```python
from build123d import *

# Parameters (mm, degrees)
SKETCH1_W           = 148
SKETCH1_H           = 106
BOSS_EXTRUDE1_DEPTH = 8
CUT_EXTRUDE1_REACH  = 93.373
SKETCH3_R           = 1.65
CUT_EXTRUDE2_DEPTH  = 130.52219887
SKETCH5_R           = 1.65
CUT_EXTRUDE3_DEPTH  = 10
SKETCH6_R           = 1.65
CUT_EXTRUDE4_DEPTH  = 10


with BuildPart() as part:
    # Sketch1 → Boss-Extrude1 (new body)
    with BuildSketch(Plane.XY):
        Rectangle(SKETCH1_W, SKETCH1_H)
    extrude(amount=-BOSS_EXTRUDE1_DEPTH)

    # Sketch2 → Cut-Extrude1 (cut, up to next)
    with BuildSketch(Plane.XY, mode=Mode.PRIVATE) as cut_extrude1_sk1:
        with BuildLine():
            ThreePointArc((60.25, 33.75), (59.373475383, 36.872498999), (57, 39.082682252))
            Line((57, 39.082682252), (57, -39.082682252))
            ThreePointArc((57, -39.082682252), (59.373475383, -36.872498999), (60.25, -33.75))
            Line((60.25, -33.75), (60.25, 33.75))
        make_face()
    cut_extrude1_tool1 = extrude(cut_extrude1_sk1.sketch, amount=-CUT_EXTRUDE1_REACH, mode=Mode.PRIVATE) & part.part
    # Sketch2 → Cut-Extrude1 (cut, up to next)
    with BuildSketch(Plane.XY, mode=Mode.PRIVATE) as cut_extrude1_sk2:
        with BuildLine():
            ThreePointArc((-54.25, 39.75), (-55.66490397, 39.580784403), (-57, 39.082682252))
            Line((-57, 39.082682252), (-57, -39.082682252))
            ThreePointArc((-57, -39.082682252), (-55.66490397, -39.580784403), (-54.25, -39.75))
            Line((-54.25, -39.75), (54.25, -39.75))
            ThreePointArc((54.25, -39.75), (55.66490397, -39.580784403), (57, -39.082682252))
            Line((57, -39.082682252), (57, 39.082682252))
            ThreePointArc((57, 39.082682252), (55.66490397, 39.580784403), (54.25, 39.75))
            Line((54.25, 39.75), (-54.25, 39.75))
        make_face()
    cut_extrude1_tool2 = extrude(cut_extrude1_sk2.sketch, amount=-CUT_EXTRUDE1_REACH, mode=Mode.PRIVATE) & part.part
    # Sketch2 → Cut-Extrude1 (cut, up to next)
    with BuildSketch(Plane.XY, mode=Mode.PRIVATE) as cut_extrude1_sk3:
        with BuildLine():
            Line((-57, -39.082682252), (-57, 39.082682252))
            ThreePointArc((-57, 39.082682252), (-59.373475383, 36.872498999), (-60.25, 33.75))
            Line((-60.25, 33.75), (-60.25, -33.75))
            ThreePointArc((-60.25, -33.75), (-59.373475383, -36.872498999), (-57, -39.082682252))
        make_face()
    cut_extrude1_tool3 = extrude(cut_extrude1_sk3.sketch, amount=-CUT_EXTRUDE1_REACH, mode=Mode.PRIVATE) & part.part
    # Sketch2 → Cut-Extrude1 (cut, up to next)
    with BuildSketch(Plane.XY, mode=Mode.PRIVATE) as cut_extrude1_sk4:
        with BuildLine():
            ThreePointArc((59.1, 46), (57, 48.1), (54.9, 46))
            Line((54.9, 46), (57, 46))
            Line((57, 46), (57, 43.9))
            ThreePointArc((57, 43.9), (58.48492424, 44.51507576), (59.1, 46))
        make_face()
    cut_extrude1_tool4 = extrude(cut_extrude1_sk4.sketch, amount=-CUT_EXTRUDE1_REACH, mode=Mode.PRIVATE) & part.part
    # Sketch2 → Cut-Extrude1 (cut, up to next)
    with BuildSketch(Plane.XY, mode=Mode.PRIVATE) as cut_extrude1_sk5:
        with BuildLine():
            Line((57, 46), (54.9, 46))
            ThreePointArc((54.9, 46), (55.51507576, 44.51507576), (57, 43.9))
            Line((57, 43.9), (57, 46))
        make_face()
    cut_extrude1_tool5 = extrude(cut_extrude1_sk5.sketch, amount=-CUT_EXTRUDE1_REACH, mode=Mode.PRIVATE) & part.part
    # Sketch2 → Cut-Extrude1 (cut, up to next)
    with BuildSketch(Plane.XY, mode=Mode.PRIVATE) as cut_extrude1_sk6:
        with BuildLine():
            ThreePointArc((59.1, 46), (57, 48.1), (54.9, 46))
            Line((54.9, 46), (57, 46))
            Line((57, 46), (57, 43.9))
            ThreePointArc((57, 43.9), (58.48492424, 44.51507576), (59.1, 46))
        make_face()
    cut_extrude1_tool6 = extrude(cut_extrude1_sk6.sketch, amount=-CUT_EXTRUDE1_REACH, mode=Mode.PRIVATE) & part.part
    # Sketch2 → Cut-Extrude1 (cut, up to next)
    with BuildSketch(Plane.XY, mode=Mode.PRIVATE) as cut_extrude1_sk7:
        with BuildLine():
            Line((57, 46), (54.9, 46))
            ThreePointArc((54.9, 46), (55.51507576, 44.51507576), (57, 43.9))
            Line((57, 43.9), (57, 46))
        make_face()
    cut_extrude1_tool7 = extrude(cut_extrude1_sk7.sketch, amount=-CUT_EXTRUDE1_REACH, mode=Mode.PRIVATE) & part.part
    # Sketch2 → Cut-Extrude1 (cut, up to next)
    with BuildSketch(Plane.XY, mode=Mode.PRIVATE) as cut_extrude1_sk8:
        with BuildLine():
            Line((-57, 43.9), (-57, 46))
            Line((-57, 46), (-54.9, 46))
            ThreePointArc((-54.9, 46), (-58.48492424, 47.48492424), (-57, 43.9))
        make_face()
    cut_extrude1_tool8 = extrude(cut_extrude1_sk8.sketch, amount=-CUT_EXTRUDE1_REACH, mode=Mode.PRIVATE) & part.part
    # Sketch2 → Cut-Extrude1 (cut, up to next)
    with BuildSketch(Plane.XY, mode=Mode.PRIVATE) as cut_extrude1_sk9:
        with BuildLine():
            Line((-54.9, 46), (-57, 46))
            Line((-57, 46), (-57, 43.9))
            ThreePointArc((-57, 43.9), (-55.51507576, 44.51507576), (-54.9, 46))
        make_face()
    cut_extrude1_tool9 = extrude(cut_extrude1_sk9.sketch, amount=-CUT_EXTRUDE1_REACH, mode=Mode.PRIVATE) & part.part
    # Sketch2 → Cut-Extrude1 (cut, up to next)
    with BuildSketch(Plane.XY, mode=Mode.PRIVATE) as cut_extrude1_sk10:
        with BuildLine():
            Line((-57, 43.9), (-57, 46))
            Line((-57, 46), (-54.9, 46))
            ThreePointArc((-54.9, 46), (-58.48492424, 47.48492424), (-57, 43.9))
        make_face()
    cut_extrude1_tool10 = extrude(cut_extrude1_sk10.sketch, amount=-CUT_EXTRUDE1_REACH, mode=Mode.PRIVATE) & part.part
    # Sketch2 → Cut-Extrude1 (cut, up to next)
    with BuildSketch(Plane.XY, mode=Mode.PRIVATE) as cut_extrude1_sk11:
        with BuildLine():
            Line((-54.9, 46), (-57, 46))
            Line((-57, 46), (-57, 43.9))
            ThreePointArc((-57, 43.9), (-55.51507576, 44.51507576), (-54.9, 46))
        make_face()
    cut_extrude1_tool11 = extrude(cut_extrude1_sk11.sketch, amount=-CUT_EXTRUDE1_REACH, mode=Mode.PRIVATE) & part.part
    # Sketch2 → Cut-Extrude1 (cut, up to next)
    with BuildSketch(Plane.XY, mode=Mode.PRIVATE) as cut_extrude1_sk12:
        with BuildLine():
            ThreePointArc((-54.9, -46), (-55.51507576, -44.51507576), (-57, -43.9))
            Line((-57, -43.9), (-57, -46))
            Line((-57, -46), (-54.9, -46))
        make_face()
    cut_extrude1_tool12 = extrude(cut_extrude1_sk12.sketch, amount=-CUT_EXTRUDE1_REACH, mode=Mode.PRIVATE) & part.part
    # Sketch2 → Cut-Extrude1 (cut, up to next)
    with BuildSketch(Plane.XY, mode=Mode.PRIVATE) as cut_extrude1_sk13:
        with BuildLine():
            Line((-57, -46), (-57, -43.9))
            ThreePointArc((-57, -43.9), (-58.48492424, -47.48492424), (-54.9, -46))
            Line((-54.9, -46), (-57, -46))
        make_face()
    cut_extrude1_tool13 = extrude(cut_extrude1_sk13.sketch, amount=-CUT_EXTRUDE1_REACH, mode=Mode.PRIVATE) & part.part
    # Sketch2 → Cut-Extrude1 (cut, up to next)
    with BuildSketch(Plane.XY, mode=Mode.PRIVATE) as cut_extrude1_sk14:
        with BuildLine():
            ThreePointArc((-54.9, -46), (-55.51507576, -44.51507576), (-57, -43.9))
            Line((-57, -43.9), (-57, -46))
            Line((-57, -46), (-54.9, -46))
        make_face()
    cut_extrude1_tool14 = extrude(cut_extrude1_sk14.sketch, amount=-CUT_EXTRUDE1_REACH, mode=Mode.PRIVATE) & part.part
    # Sketch2 → Cut-Extrude1 (cut, up to next)
    with BuildSketch(Plane.XY, mode=Mode.PRIVATE) as cut_extrude1_sk15:
        with BuildLine():
            Line((-57, -46), (-57, -43.9))
            ThreePointArc((-57, -43.9), (-58.48492424, -47.48492424), (-54.9, -46))
            Line((-54.9, -46), (-57, -46))
        make_face()
    cut_extrude1_tool15 = extrude(cut_extrude1_sk15.sketch, amount=-CUT_EXTRUDE1_REACH, mode=Mode.PRIVATE) & part.part
    # Sketch2 → Cut-Extrude1 (cut, up to next)
    with BuildSketch(Plane.XY, mode=Mode.PRIVATE) as cut_extrude1_sk16:
        with BuildLine():
            ThreePointArc((59.1, -46), (58.48492424, -44.51507576), (57, -43.9))
            Line((57, -43.9), (57, -46))
            Line((57, -46), (54.9, -46))
            ThreePointArc((54.9, -46), (57, -48.1), (59.1, -46))
        make_face()
    cut_extrude1_tool16 = extrude(cut_extrude1_sk16.sketch, amount=-CUT_EXTRUDE1_REACH, mode=Mode.PRIVATE) & part.part
    # Sketch2 → Cut-Extrude1 (cut, up to next)
    with BuildSketch(Plane.XY, mode=Mode.PRIVATE) as cut_extrude1_sk17:
        with BuildLine():
            Line((57, -46), (57, -43.9))
            ThreePointArc((57, -43.9), (55.51507576, -44.51507576), (54.9, -46))
            Line((54.9, -46), (57, -46))
        make_face()
    cut_extrude1_tool17 = extrude(cut_extrude1_sk17.sketch, amount=-CUT_EXTRUDE1_REACH, mode=Mode.PRIVATE) & part.part
    # Sketch2 → Cut-Extrude1 (cut, up to next)
    with BuildSketch(Plane.XY, mode=Mode.PRIVATE) as cut_extrude1_sk18:
        with BuildLine():
            ThreePointArc((59.1, -46), (58.48492424, -44.51507576), (57, -43.9))
            Line((57, -43.9), (57, -46))
            Line((57, -46), (54.9, -46))
            ThreePointArc((54.9, -46), (57, -48.1), (59.1, -46))
        make_face()
    cut_extrude1_tool18 = extrude(cut_extrude1_sk18.sketch, amount=-CUT_EXTRUDE1_REACH, mode=Mode.PRIVATE) & part.part
    # Sketch2 → Cut-Extrude1 (cut, up to next)
    with BuildSketch(Plane.XY, mode=Mode.PRIVATE) as cut_extrude1_sk19:
        with BuildLine():
            Line((57, -46), (57, -43.9))
            ThreePointArc((57, -43.9), (55.51507576, -44.51507576), (54.9, -46))
            Line((54.9, -46), (57, -46))
        make_face()
    cut_extrude1_tool19 = extrude(cut_extrude1_sk19.sketch, amount=-CUT_EXTRUDE1_REACH, mode=Mode.PRIVATE) & part.part
    add(cut_extrude1_tool1.solids().sort_by_distance((58.595694, 0, 0))[0], mode=Mode.SUBTRACT)
    add(cut_extrude1_tool2.solids().sort_by_distance((0, 0, 0))[0], mode=Mode.SUBTRACT)
    add(cut_extrude1_tool3.solids().sort_by_distance((-58.595694, 0, 0))[0], mode=Mode.SUBTRACT)
    add(cut_extrude1_tool4.solids().sort_by_distance((57.297089, 46.297089, 0))[0], mode=Mode.SUBTRACT)
    add(cut_extrude1_tool5.solids().sort_by_distance((56.108732, 45.108732, 0))[0], mode=Mode.SUBTRACT)
    add(cut_extrude1_tool6.solids().sort_by_distance((57.297089, 46.297089, 0))[0], mode=Mode.SUBTRACT)
    add(cut_extrude1_tool7.solids().sort_by_distance((56.108732, 45.108732, 0))[0], mode=Mode.SUBTRACT)
    add(cut_extrude1_tool8.solids().sort_by_distance((-57.297089, 46.297089, 0))[0], mode=Mode.SUBTRACT)
    add(cut_extrude1_tool9.solids().sort_by_distance((-56.108732, 45.108732, 0))[0], mode=Mode.SUBTRACT)
    add(cut_extrude1_tool10.solids().sort_by_distance((-57.297089, 46.297089, 0))[0], mode=Mode.SUBTRACT)
    add(cut_extrude1_tool11.solids().sort_by_distance((-56.108732, 45.108732, 0))[0], mode=Mode.SUBTRACT)
    add(cut_extrude1_tool12.solids().sort_by_distance((-56.108732, -45.108732, 0))[0], mode=Mode.SUBTRACT)
    add(cut_extrude1_tool13.solids().sort_by_distance((-57.297089, -46.297089, 0))[0], mode=Mode.SUBTRACT)
    add(cut_extrude1_tool14.solids().sort_by_distance((-56.108732, -45.108732, 0))[0], mode=Mode.SUBTRACT)
    add(cut_extrude1_tool15.solids().sort_by_distance((-57.297089, -46.297089, 0))[0], mode=Mode.SUBTRACT)
    add(cut_extrude1_tool16.solids().sort_by_distance((57.297089, -46.297089, 0))[0], mode=Mode.SUBTRACT)
    add(cut_extrude1_tool17.solids().sort_by_distance((56.108732, -45.108732, 0))[0], mode=Mode.SUBTRACT)
    add(cut_extrude1_tool18.solids().sort_by_distance((57.297089, -46.297089, 0))[0], mode=Mode.SUBTRACT)
    add(cut_extrude1_tool19.solids().sort_by_distance((56.108732, -45.108732, 0))[0], mode=Mode.SUBTRACT)

    # Sketch3 → Cut-Extrude2 (cut, through all)
    with BuildSketch(Plane.XZ.offset(53)):
        with Locations(Location((-39, -4, 0), (0, 0, 270))):
            Circle(SKETCH3_R)
        with Locations(Location((0, -4, 0), (0, 0, 270))):
            Circle(SKETCH3_R)
        with Locations(Location((39, -4, 0), (0, 0, 270))):
            Circle(SKETCH3_R)
    extrude(amount=-CUT_EXTRUDE2_DEPTH, mode=Mode.SUBTRACT)

    # Sketch5 → Cut-Extrude3 (cut)
    with BuildSketch(Plane(origin=(74, 0, 0), x_dir=(0, 0, -1), z_dir=(1, 0, 0))):
        with Locations((4, 39.75)):
            Circle(SKETCH5_R)
        with Locations((4, 13.25)):
            Circle(SKETCH5_R)
        with Locations((4, -13.25)):
            Circle(SKETCH5_R)
        with Locations((4, -39.75)):
            Circle(SKETCH5_R)
    extrude(amount=-CUT_EXTRUDE3_DEPTH, mode=Mode.SUBTRACT)

    # Sketch6 → Cut-Extrude4 (cut)
    with BuildSketch(Plane.ZY.offset(74)):
        with Locations(Location((-4, 39.75, 0), (0, 0, 180))):
            Circle(SKETCH6_R)
        with Locations(Location((-4, 13.25, 0), (0, 0, 180))):
            Circle(SKETCH6_R)
        with Locations(Location((-4, -13.25, 0), (0, 0, 180))):
            Circle(SKETCH6_R)
        with Locations(Location((-4, -39.75, 0), (0, 0, 180))):
            Circle(SKETCH6_R)
    extrude(amount=-CUT_EXTRUDE4_DEPTH, mode=Mode.SUBTRACT)


solid = part.part
```
For this review, take the finished solid that the model builds, in its own axes (mm). A direction names the side the tool comes from. Round coordinates to 2 decimals unless told otherwise and drop trailing zeros. Write each loop counter-clockwise with the first axis right and the second up, starting at its lowest first coordinate (ties: lowest second). Pieces come first, ordered by that corner, then holes. Notation, with made-up numbers: (28, -12) - (56, -12) arc R10 cw to (56, -1) - close; hole circle Ø9 at (43.5, 19.25). An arc over 180 degrees is marked (long way). Use CSV: the item, a comma, the result in double quotes.
1) Clearance check with flat-ended pins moving along their axes: pin 1 Ø3 at (x, z) = (39, -4) entering from +Y; pin 2 Ø2 at (y, z) = (-13.25, -4) entering from -X; pin 3 Ø2 at (y, z) = (-39.75, -4) entering from +X. State where each tip first meets the part, or that it passes through.
Conclusion:
pin 1,"passes through"
pin 2,"stops at x = -64"
pin 3,"stops at x = 64"
2) Add section D-D on z = -4. Count the separate pieces of the cut face and the enclosed holes in it, and give its area (3 significant figures).
Conclusion:
separate pieces,"6"
enclosed holes,"4"
area,"5,560 mm^2"
3) Add section B-B on x = 12. Write out the cut boundary in (y, z).
Conclusion:
outline,"(-53, -8) - (-39.75, -8) - (-39.75, 0) - (-53, 0) - close; (39.75, -8) - (53, -8) - (53, 0) - (39.75, 0) - close"
4) Add section A-A on y = 13.25. Write out the cut boundary in (x, z), and give its area (3 significant figures).
Conclusion:
outline,"(-74, -8) - (-60.25, -8) - (-60.25, 0) - (-74, 0) - (-74, -2.35) - (-64, -2.35) - (-64, -5.65) - (-74, -5.65) - close; (60.25, -8) - (74, -8) - (74, -5.65) - (64, -5.65) - (64, -2.35) - (74, -2.35) - (74, 0) - (60.25, 0) - close"
area,"154 mm^2"
5) Wall thickness on line 1 along Y through (x, z) = (71, -4); line 2 along Y through (x, z) = (-57, -5); line 3 along Y through (x, z) = (18.5, -2.5): over which ranges is each line inside the solid? List them lowest first. Write a range as from..to.
Conclusion:
line 1,"y = -53..-41.4, -38.1..-14.9, -11.6..11.6, 14.9..38.1, 41.4..53"
line 2,"y = -53..-48.1, -43.9..-39.08, 39.08..43.9, 48.1..53"
line 3,"y = -53..-39.75, 39.75..53"
6) Add section C-C on x = -39. Write out the cut boundary in (y, z), and give its area (3 significant figures).
Conclusion:
outline,"(-53, -8) - (-39.75, -8) - (-39.75, -5.65) - (-53, -5.65) - close; (-53, -2.35) - (-39.75, -2.35) - (-39.75, 0) - (-53, 0) - close; (39.75, -8) - (53, -8) - (53, -5.65) - (39.75, -5.65) - close; (39.75, -2.35) - (53, -2.35) - (53, 0) - (39.75, 0) - close"
area,"125 mm^2"
7) For faces 5 (the flat face through (-60.25, 0, -4)), 6 (the cylindrical face through (69.07, 41.386, -3.785)), 7 (the flat face through (-1, -46, 0)), 8 (the cylindrical face through (-69.07, -41.386, -3.785)), list the 3-axis set-ups (+Z, -Z, +X, -X, +Y, -Y) from which the entire face can be reached by the end or side of a thin tool; tool diameter is ignored.
Conclusion:
face 5,"+Z, -Z"
face 6,"+X"
face 7,"+Z, +X, -X, +Y, -Y"
face 8,"-X"
8) The part is to be moulded in two halves that separate along X. For faces 1 (the cylindrical face through (-37.61, 46.28, -4.89)), 2 (the flat face through (64, -40, -4)), 3 (the cylindrical face through (0.07, -46.47, -2.35)), 4 (the cylindrical face through (69.07, -13.18, -2.35)), say which applies: pulls with the +X half, pulls with the -X half, needs draft (parallel to the pull), parting line crosses it, or undercut.
Conclusion:
face 1,"undercut"
face 2,"pulls with the +X half"
face 3,"undercut"
face 4,"needs draft"
